from build123d import *

# Parameters (mm, degrees)
SKETCH1_W           = 22.6
SKETCH1_H           = 23
BOSS_EXTRUDE1_DEPTH = 12
SKETCH2_R           = 6
BOSS_EXTRUDE2_DEPTH = 4
SKETCH3_R           = 2.4
BOSS_EXTRUDE3_DEPTH = 2.5
SKETCH4_W           = 12
SKETCH4_H           = 5
SKETCH4_R           = 1
BOSS_EXTRUDE4_DEPTH = 2.3


with BuildPart() as part:
    # Sketch1 → Boss-Extrude1 (new body)
    with BuildSketch(Plane(origin=(0, 0, 0), x_dir=(0, 0, -1), z_dir=(1, 0, 0))):
        with Locations((11.3, 11.5)):
            Rectangle(SKETCH1_W, SKETCH1_H)
    extrude(amount=BOSS_EXTRUDE1_DEPTH)

    # Sketch2 → Boss-Extrude2 (add)
    with BuildSketch(Plane(origin=(0, 23, 0), x_dir=(1, 0, 0), z_dir=(0, 1, 0))):
        with Locations(Location((6, 6, 0), (0, 0, 270))):
            Circle(SKETCH2_R)
    extrude(amount=BOSS_EXTRUDE2_DEPTH)

    # Sketch3 → Boss-Extrude3 (add)
    with BuildSketch(Plane(origin=(0, 27, 0), x_dir=(1, 0, 0), z_dir=(0, 1, 0))):
        with Locations(Location((6, 6, 0), (0, 0, 270))):
            Circle(SKETCH3_R)
    extrude(amount=BOSS_EXTRUDE3_DEPTH)

    # Sketch4 → Boss-Extrude4 (add)
    # profile 1 of 2: a face of its own
    with BuildSketch(Plane(origin=(0, 16.5, 0), x_dir=(1, 0, 0), z_dir=(0, 1, 0))):
        with Locations((6, -2.5)):
            Rectangle(SKETCH4_W, SKETCH4_H)
        with Locations(Location((6, -3, 0), (0, 0, 270))):
            Circle(SKETCH4_R, mode=Mode.SUBTRACT)
    # profile 2 of 2: a face of its own
    with BuildSketch(Plane(origin=(0, 16.5, 0), x_dir=(1, 0, 0), z_dir=(0, 1, 0))):
        with Locations((6, 25.1)):
            Rectangle(SKETCH4_W, SKETCH4_H)
        with Locations(Location((6, 25.6, 0), (0, 0, 270))):
            Circle(SKETCH4_R, mode=Mode.SUBTRACT)
    extrude(amount=BOSS_EXTRUDE4_DEPTH)


solid = part.part
Part model, mm, in its own coordinate system. A direction names the side the tool comes from. Give positions to 0.01 mm unless a question says otherwise; leave off trailing zeros. Order: outer loops, then holes, each group sorted by start corner. A loop starts at its lowest first (then second) coordinate and runs counter-clockwise, first axis right, second up. Notation, with made-up numbers: (-2.5, 29.25) - (9.5, 29.25) arc R16 cw to (9.5, 59.25) - close; hole circle Ø6 at (48.5, 5). An arc over 180 degrees is marked (long way). Use a Markdown table: item, result.
1) Saw through at D-D on z = -2. List the corners of the cut face in (x, y), plus the area to 3 significant figures.
Checked values:
| item | result |
|---|---|
| outline | (0, 0) - (12, 0) - (12, 23) - (10.47, 23) - (10.47, 27) - (1.53, 27) - (1.53, 23) - (0, 23) - close |
| area | 312 mm² |
2) Saw through at C-C on x = 10.5. List the corners of the cut face in (y, z), plus the area to 3 significant figures.
Checked values:
| item | result |
|---|---|
| outline | (0, -22.6) - (16.5, -22.6) - (16.5, -27.6) - (18.8, -27.6) - (18.8, -22.6) - (23, -22.6) - (23, -9.97) - (27, -9.97) - (27, -2.03) - (23, -2.03) - (23, 0) - (18.8, 0) - (18.8, 5) - (16.5, 5) - (16.5, 0) - (0, 0) - close |
| area | 575 mm² |
3) Saw through at B-B on y = 17.75. List the corners of the cut face in (x, z).
Checked values:
| item | result |
|---|---|
| outline | (0, -27.6) - (12, -27.6) - (12, 5) - (0, 5) - close; hole circle Ø2 at (6, -25.6); hole circle Ø2 at (6, 3) |
4) 3-axis set-ups, long thin cutter, end or side, ignore diameter. For faces 4 (the flat face through (6, 16.5, 1)), 5 (the flat face through (6, 16.5, -24)), 6 (the flat face through (1, 23, -1)): which of +Z, -Z, +X, -X, +Y, -Y reach the whole face in a straight line?
Checked values:
| item | result |
|---|---|
| face 4 | +Z, +X, -X, -Y |
| face 5 | -Z, +X, -X, -Y |
| face 6 | +Z, -X, +Y |
5) Two-plate mould, pull along X, no slides. Class faces 1 (the cylindrical face through (6.3, 17.634, -24.646)), 2 (the cylindrical face through (6.106, 28.232, -8.398)), 3 (the flat face through (11, 23, -1)): +X half, -X half, draft (parallel to the pull), parting line (faces both ways), or undercut.
Checked values:
| item | result |
|---|---|
| face 1 | undercut |
| face 2 | parting line |
| face 3 | draft |
6) Saw through at A-A on z = 3. List the corners of the cut face in (x, y).
Checked values:
| item | result |
|---|---|
| outline | (0, 16.5) - (5, 16.5) - (5, 18.8) - (0, 18.8) - close; (7, 16.5) - (12, 16.5) - (12, 18.8) - (7, 18.8) - close |
7) Flat gauge pins, fed straight in: P1, Ø4, axis at x = 7, z = 3, coming from the -Y side; P2, Ø1.8, axis at x = 3.5, z = -3, coming from the +Y side; P3, Ø4, axis at x = 9, z = -24.5, coming from the +Y side. Where does each tip first touch, or does it go through?
Checked values:
| item | result |
|---|---|
| P1 | y = 16.5 |
| P2 | y = 27 |
| P3 | y = 23 |
8) Probe L1, parallel to X at y = 17.3, z = -25.6; L2, parallel to Z at x = 2.75, y = 8.5; L3, parallel to Y at x = 9.75, z = -3.5. List the from-to ranges inside material, lowest first. Write a range as from..to.
Checked values:
| item | result |
|---|---|
| L1 | 0..5, 7..12 |
| L2 | -22.6..0 |
| L3 | 0..27 |
